from build123d import *

# Parameters (mm, degrees)
SKETCH1_W                = 7
SKETCH1_H                = 4
BOSS_EXTRUDE1_DEPTH      = 2.5
SKETCH2_R                = 0.75
CUT_EXTRUDE1_DEPTH       = 0.2
SKETCH3_W                = 0.3
SKETCH3_H                = 3.7
BOSS_EXTRUDE2_DEPTH      = 3.5
BOSS_EXTRUDE2_DEPTH_BACK = 3.5
CUT_EXTRUDE2_DEPTH       = 3.5
CUT_EXTRUDE2_DEPTH_BACK  = 1


with BuildPart() as part:
    # Sketch1 → Boss-Extrude1 (new body)
    with BuildSketch(Plane.XY):
        Rectangle(SKETCH1_W, SKETCH1_H)
    extrude(amount=BOSS_EXTRUDE1_DEPTH)

    # Sketch2 → Cut-Extrude1 (cut)
    with BuildSketch(Plane.XY.offset(2.5)):
        with Locations((-1.27, 0.2)):
            Circle(SKETCH2_R)
        with Locations((1.27, 0.2)):
            Circle(SKETCH2_R)
    extrude(amount=-CUT_EXTRUDE1_DEPTH, mode=Mode.SUBTRACT)

    # Sketch3 → Boss-Extrude2 (add, two sides)
    with BuildSketch(Plane(origin=(0, 0, 0), x_dir=(0, 0, -1), z_dir=(1, 0, 0))) as boss_extrude2_sk:
        with Locations((-1.05, -3.85)):
            Rectangle(SKETCH3_W, SKETCH3_H)
    extrude(amount=BOSS_EXTRUDE2_DEPTH)
    extrude(boss_extrude2_sk.sketch, amount=-BOSS_EXTRUDE2_DEPTH_BACK)

    # Sketch4 → Cut-Extrude2 (cut, two sides)
    with BuildSketch(Plane.XY) as cut_extrude2_sk:
        Polygon((-2.79, -6.068420348), (-2.79, -4.468420348), (-3.020094846, -4.468420348), (-3.020094846, -3.968420348), (-2.79, -3.968420348), (-2.79, -2), (-4.136093054, -2), (-4.136093054, -6.068420348), align=None)
        Polygon((-2.29, -6.068420348), (-2.29, -4.468420348), (-2.059905154, -4.468420348), (-2.059905154, -3.968420348), (-2.29, -3.968420348), (-2.29, -2), (-1.52, -2), (-1.52, -3.968420348), (-1.750094846, -3.968420348), (-1.750094846, -4.468420348), (-1.52, -4.468420348), (-1.52, -6.068420348), align=None)
        Polygon((-1.02, -2), (1.02, -2), (1.02, -3.968420348), (0.789905154, -3.968420348), (0.789905154, -4.468420348), (1.02, -4.468420348), (1.02, -6.068420348), (-1.02, -6.068420348), (-1.02, -4.468420348), (-0.789905154, -4.468420348), (-0.789905154, -3.968420348), (-1.02, -3.968420348), align=None)
        Polygon((4.136093054, -6.068420348), (2.79, -6.068420348), (2.79, -4.468420348), (3.020094846, -4.468420348), (3.020094846, -3.968420348), (2.79, -3.968420348), (2.79, -2), (4.136093054, -2), align=None)
        Polygon((1.52, -6.068420348), (1.52, -4.468420348), (1.750094846, -4.468420348), (1.750094846, -3.968420348), (1.52, -3.968420348), (1.52, -2), (2.29, -2), (2.29, -3.968420348), (2.059905154, -3.968420348), (2.059905154, -4.468420348), (2.29, -4.468420348), (2.29, -6.068420348), align=None)
    extrude(amount=CUT_EXTRUDE2_DEPTH, mode=Mode.SUBTRACT)
    extrude(cut_extrude2_sk.sketch, amount=-CUT_EXTRUDE2_DEPTH_BACK, mode=Mode.SUBTRACT)


solid = part.part
The listing builds one solid part. Answer for the finished solid, in the listing's coordinates (mm). A direction names the side the tool comes from. Round coordinates to 2 decimals unless told otherwise and drop trailing zeros. Loops run counter-clockwise (first coordinate to the right, second up) from the corner with the lowest first, then second, coordinate; pieces in that order, holes last. Notation, with made-up numbers: M -9.75,70 L 36.25,70 A21 ccw 36.25,92 Z; hole C 18.5,68 d1. An arc over 180 degrees is marked long. Write each question's results on one line, items separated by ' | '. Start each with the question number.
1) Straight lines are drawn through the part: probe 1 along Y at (x, z) = (1.27, 2.4); probe 2 along Y at (x, z) = (-0.5, 0.6); probe 3 along Z at (x, y) = (1, 0.25). For each, find the intervals that lie inside material, in ascending order.
2) This flat-tipped pin is pushed along its axis until it touches: pin 1 (0.8 mm diameter, centred on x = 2.5, y = -3.5, fed in from -Z). Where does it stop, or does it pass through?
3) Find section C-C on y = 0.2. Write down the section's boundary in (x, z).
4) Find section D-D on z = 1.6. Write down the section's boundary in (x, y).
5) Find section B-B on x = -1.27. Write down the section's boundary in (y, z).
6) Which of the six approach directions +Z, -Z, +X, -X, +Y, -Y give full straight-line access (tool end or side, diameter ignored) to faces 1 (the flat face through (-1, 0, 2.3)), 2 (the flat face through (2.5, -3.9, 0.9)), 3 (the flat face through (2.5, -3.9, 1.2)), 4 (the flat face through (0, 2, 1))?
7) Determine the mould class of faces 5 (the flat face through (1.3, -3.9, 1.2)), 6 (the flat face through (1, 0, 2.3)), 7 (the flat face through (3.5, 0, 1)) for opening direction X: pulls with the +X half, pulls with the -X half, needs draft (parallel to the pull), parting line crosses it, or undercut.
8) Find section A-A on y = -3. Write down the section's boundary in (x, z).
Final values:
1) probe 1: -2 to -0.55, 0.95 to 2 | probe 2: -2 to 2 | probe 3: 0 to 2.3
2) pin 1: z = 0.9
3) outline: M -3.5,0 L 3.5,0 L 3.5,2.5 L 2.02,2.5 L 2.02,2.3 L 0.52,2.3 L 0.52,2.5 L -0.52,2.5 L -0.52,2.3 L -2.02,2.3 L -2.02,2.5 L -3.5,2.5 Z
4) outline: M -3.5,-2 L 3.5,-2 L 3.5,2 L -3.5,2 Z
5) outline: M -5.7,0.9 L -2,0.9 L -2,0 L 2,0 L 2,2.5 L 0.95,2.5 L 0.95,2.3 L -0.55,2.3 L -0.55,2.5 L -2,2.5 L -2,1.2 L -5.7,1.2 Z
6) face 1: +Z | face 2: -Z, +X, -X, -Y | face 3: +Z, +X, -X, -Y | face 4: +Z, -Z, +X, -X, +Y
7) face 5: needs draft | face 6: undercut | face 7: pulls with the +X half
8) outline: M -2.79,0.9 L -2.29,0.9 L -2.29,1.2 L -2.79,1.2 Z; M -1.52,0.9 L -1.02,0.9 L -1.02,1.2 L -1.52,1.2 Z; M 1.02,0.9 L 1.52,0.9 L 1.52,1.2 L 1.02,1.2 Z; M 2.29,0.9 L 2.79,0.9 L 2.79,1.2 L 2.29,1.2 Z
